CAD build for the part. Positions are in the model's coordinates, mm. Round coordinates to 2 decimals unless told otherwise and drop trailing zeros. Order: outer loops, then holes, each group sorted by start corner. A loop starts at its lowest first (then second) coordinate and runs counter-clockwise, first axis right, second up. Notation, with made-up numbers: M 58,2 L 65,2 A28 cw 65,41 Z; hole C 14,22 d2. An arc over 180 degrees is marked long. Answer as a JSON object with one key per item and string values. Group by question number.
Autodesk Inventor part; units mm, degrees
ref_plane "YZ Plane" through (0, 0, 0) normal (1, 0, 0) x (0, 1, 0)
ref_plane "XZ Plane" through (0, 0, 0) normal (0, 1, 0) x (-1, 0, 0)
ref_plane "XY Plane" through (0, 0, 0) normal (0, 0, 1) x (1, 0, 0)
sketch "Szkic1" plane through (0, 0, 0) normal (0, 0, 1) x (1, 0, 0)
  line L0 (0, -39.2) -> (0, 39.2)
  line L1 (-63, 0) -> (63, 0)
  line L2 (-45, -28) -> (45, -28)
  line L3 (45, -28) -> (45, 28)
  line L4 (45, 28) -> (-45, 28)
  line L5 (-45, 28) -> (-45, -28)
  line L6 (-45, -28) -> (45, 28) construction
  line L7 (45, -28) -> (-45, 28) construction
  point P0 (0, 0)
  dimension "d0" = 90
  dimension "d1" = 56
extrude "Wyciągnięcie proste1" add sketch "Szkic1" along normal blind 3
sketch "Szkic2" plane through (45, -28, 0) normal (1, 0, 0) x (0, 0, -1)
  line L0 (-3, 0) -> (-3, 56)
  line L1 (-3, 56) -> (0, 50.8038)
  line L2 (0, 0) -> (0, 56)
  line L3 (0, 0) -> (0, 56)
  line L4 (0, 56) -> (-3, 56)
  line L5 (-3, 0) -> (-3, 56)
  line L6 (0, 0) -> (-3, 0)
  point P0 (0, 28)
  dimension "d4" = 30
extrude "Wyciągnięcie proste2" cut sketch "Szkic2" against normal blind 90 contours L4 L2 L1
sketch "Szkic3" plane through (0, 0, 3) normal (0, 0, 1) x (1, 0, 0)
  line L0 (-45, -28) -> (45, -28)
  line L1 (45, -28) -> (45, 28)
  line L2 (45, 28) -> (-45, 28)
  line L3 (-45, 28) -> (-45, -28)
  point P0 (0, 0)
  point P1 (40.5, 5.5)
  point P2 (40.5, -24.5)
  dimension "d7" = 4.5
  dimension "d8" = 4.5
  dimension "d9" = 3.5
  dimension "d10" = 30
hole "Otwór1" at (40.5, 5.5, 3) at (40.5, -24.5, 3) direction (0, 0, -1) diameter 3 depth 3
mirror "Odbij1" about plane through (0, 0, 0) normal (1, 0, 0) of "Otwór1"
properties part number "obciążenie_dół" material "Stal"
Item 1: Drill centre lines: line 1 (X direction, y = 5.5, z = 2.3); line 2 (Y direction, x = 40.5, z = 0.6); line 3 (Y direction, x = 40.5, z = 2.3). Where is each one in solid material? Low to high. Write a range as [from, to].
Item 2: Cut at C-C, the plane z = 1.6. Give the cut face in (x, y), and give its area (3 significant figures).
Item 3: Two-plate mould, pull along X, no slides. Class faces 1 (the face through (-39.036, 5.825, 1.479)), 2 (the face through (-1, -2, 0)), 3 (the face through (-45, 0, 1)): +X half, -X half, draft (parallel to the pull), parting line (faces both ways), or undercut.
Item 4: Cut at A-A, the plane x = -40.5. Give the cut face in (y, z), and give its area (3 significant figures).
Item 5: Flat gauge pin, fed straight in: pin 1 Ø1.5 at (x, z) = (10, 1) entering from +Y. Where does the tip first touch, or does it go through?
Item 6: Cut at D-D, the plane x = 16.5. Give the cut face in (y, z), and give its area (3 significant figures).
Item 7: Cut at B-B, the plane y = 5.5. Give the cut face in (x, z).
Response values:
{
 "1": {"line 1": "[-45, -42], [-39, 39], [42, 45]", "line 2": "[-28, -26], [-23, 4], [7, 23.84]", "line 3": "[-28, -26], [-23, 4], [7, 26.79]"},
 "2": {"outline": "M -45,-28 L 45,-28 L 45,25.58 L -45,25.58 Z; hole C -40.5,-24.5 d3; hole C -40.5,5.5 d3; hole C 40.5,-24.5 d3; hole C 40.5,5.5 d3", "area": "4,790 mm^2"},
 "3": {"face 1": "undercut", "face 2": "draft", "face 3": "-X half"},
 "4": {"outline": "M -28,0 L -26,0 L -26,3 L -28,3 Z; M -23,0 L 4,0 L 4,3 L -23,3 Z; M 7,0 L 22.8,0 L 28,3 L 7,3 Z", "area": "142 mm^2"},
 "5": {"pin 1": "y = 25.83"},
 "6": {"outline": "M -28,0 L 22.8,0 L 28,3 L -28,3 Z", "area": "160 mm^2"},
 "7": {"outline": "M -45,0 L -42,0 L -42,3 L -45,3 Z; M -39,0 L 39,0 L 39,3 L -39,3 Z; M 42,0 L 45,0 L 45,3 L 42,3 Z"}
}
